CAD build for the part. Positions are in the model's coordinates, mm. Give positions to 0.01 mm unless a question says otherwise; leave off trailing zeros. Write each loop counter-clockwise with the first axis right and the second up, starting at its lowest first coordinate (ties: lowest second). Pieces come first, ordered by that corner, then holes. Notation, with made-up numbers: M 22,-28 L 80,-28 A18 ccw 80,-21 Z; hole C 7.5,69 d7. An arc over 180 degrees is marked long. One line per question, with ' | ' between items. Start each with the question number.
1. Flat gauge pin, fed straight in: pin 1 (3 mm diameter, centred on x = -38.1, z = 247.65, fed in from -Y). Where does the tip first touch, or does it go through?
2. Wall check: L1, parallel to Z at x = 25.5, y = 5; L2, parallel to Z at x = 12.7, y = 3.75; L3, parallel to Z at x = 8.5, y = 3. Give the ranges that are in metal, low to high.
3. Cut at A-A, the plane z = 107.95. Write the cut outline in (x, y), then the cut area to 3 significant figures.
4. Cut at B-B, the plane y = 3. Count the separate pieces of the cut face and the enclosed holes in it, then the cut area to 3 significant figures.
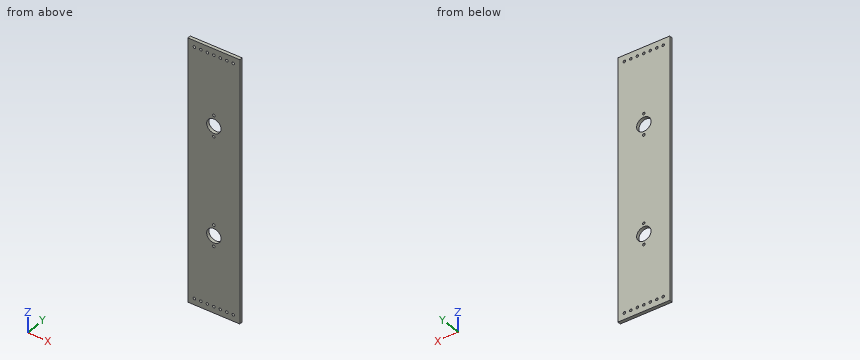
Autodesk Inventor part; units mm, degrees
ref_plane "YZ Plane" through (0, 0, 0) normal (1, 0, 0) x (0, 1, 0)
ref_plane "XZ Plane" through (0, 0, 0) normal (0, 1, 0) x (-1, 0, 0)
ref_plane "XY Plane" through (0, 0, 0) normal (0, 0, 1) x (1, 0, 0)
sketch "Sketch1" plane through (0, 0, 0) normal (0, 1, 0) x (-1, 0, 0)
  line L0 (-50.8, -260.35) -> (50.8, -260.35)
  line L1 (50.8, -260.35) -> (50.8, 260.35)
  line L2 (50.8, 260.35) -> (-50.8, 260.35)
  line L3 (-50.8, 260.35) -> (-50.8, -260.35)
  line L4 (-50.8, -260.35) -> (50.8, 260.35) construction
  line L5 (50.8, -260.35) -> (-50.8, 260.35) construction
  point P0 (0, 0)
  dimension "d0" = 101.6
  dimension "d1" = 520.7
extrude "Extrusion1" add sketch "Sketch1" along normal blind 6.35
sketch "Sketch2" plane through (0, 6.35, 0) normal (0, 1, 0) x (1, 0, 0)
  circle A0 centre (0, -107.95) radius 14.097
  circle A1 centre (0, 107.95) radius 14.097
  line L0 (0, -107.95) -> (0, 107.95) construction
  circle A2 centre (0, -107.95) radius 63.5 construction
  circle A3 centre (0, 107.95) radius 63.5 construction
  circle A4 centre (-107.4015, 0) radius 57.15 construction
  circle A5 centre (0, 44.5491) radius 14.097
  point P0 (0, 0)
  point P1 (0, 0)
  point P2 (0, -44.45)
  point P3 (0, 44.45)
  dimension "d7" = 127
  dimension "d8" = 127
  dimension "d5" = 28.194
  dimension "d9" = 88.9
  dimension "d10" = 114.3
  dimension "d12" = 152.4991
extrude "Extrusion2" cut sketch "Sketch2" against normal blind 6.35 contours A0 | A1
sketch "Sketch3" plane through (0, 6.35, 0) normal (0, 1, 0) x (1, 0, 0)
  line L0 (-50.8, -260.35) -> (50.8, -260.35)
  line L1 (-50.8, 260.35) -> (-50.8, -260.35)
  line L2 (-50.8, 260.35) -> (-50.8, -260.35) construction
  line L3 (-50.8, 0) -> (50.8, 0) construction
  line L4 (50.8, -260.35) -> (50.8, 260.35) construction
  point P0 (0, 0)
  point P1 (-38.1, -247.65)
  point P2 (-25.4, -247.65)
  point P3 (-12.7, -247.65)
  point P4 (0, -247.65)
  point P5 (12.7, -247.65)
  point P6 (25.4, -247.65)
  point P7 (38.1, -247.65)
  point P8 (-38.1, 247.65)
  point P9 (-25.4, 247.65)
  point P10 (-12.7, 247.65)
  point P11 (0, 247.65)
  point P12 (12.7, 247.65)
  point P13 (25.4, 247.65)
  point P14 (38.1, 247.65)
  dimension "d15" = 12.7
  dimension "d16" = 12.7
  dimension "d19" = 12.7
hole "Hole1" at (-38.1, 6.35, 247.65) at (-25.4, 6.35, 247.65) at (-12.7, 6.35, 247.65) at (0, 6.35, 247.65) at (12.7, 6.35, 247.65) at (25.4, 6.35, 247.65) at (38.1, 6.35, 247.65) at (38.1, 6.35, -247.65) at (25.4, 6.35, -247.65) at (12.7, 6.35, -247.65) at (0, 6.35, -247.65) at (-12.7, 6.35, -247.65) at (-25.4, 6.35, -247.65) at (-38.1, 6.35, -247.65) direction (0, -1, 0) diameter 5.1054 end through all
sketch "Sketch4" plane through (0, 6.35, 0) normal (0, 1, 0) x (1, 0, 0)
  line L0 (0, -86.9315) -> (0, -128.9685) construction
  line L1 (0, 128.9685) -> (0, 86.9315) construction
  circle A0 centre (-25.4, 247.65) radius 2.5527
  circle A1 centre (0, 247.65) radius 2.5527
  circle A2 centre (25.4, 247.65) radius 2.5527
  circle A3 centre (38.1, -247.65) radius 2.5527
  circle A4 centre (12.7, -247.65) radius 2.5527
  circle A5 centre (-12.7, -247.65) radius 2.5527
  circle A6 centre (-38.1, -247.65) radius 2.5527
  circle A7 centre (-25.4, -247.65) radius 2.5527
  circle A8 centre (0, -247.65) radius 2.5527
  circle A9 centre (25.4, -247.65) radius 2.5527
  circle A10 centre (38.1, 247.65) radius 2.5527
  circle A11 centre (12.7, 247.65) radius 2.5527
  circle A12 centre (-12.7, 247.65) radius 2.5527
  circle A13 centre (-38.1, 247.65) radius 2.5527
  circle A14 centre (0, 107.95) radius 14.097
  circle A15 centre (0, -107.95) radius 14.097
  line L2 (-50.8, 260.35) -> (50.8, 260.35)
  line L3 (50.8, 260.35) -> (50.8, -260.35)
  line L4 (50.8, -260.35) -> (-50.8, -260.35)
  line L5 (-50.8, -260.35) -> (-50.8, 260.35)
  point P0 (0, 0)
  dimension "d31" = 42.037
  dimension "d32" = 42.037
hole "Hole2" at (0, 6.35, -128.9685) at (0, 6.35, -86.9315) at (0, 6.35, 86.9315) at (0, 6.35, 128.9685) direction (0, -1, 0) diameter 5.1054 end through all
properties part number "GI - 007" material "Aluminum 6061"
Here are the results:
1) pin 1: through
2) L1: -260.35 to -250.2, -245.1 to 245.1, 250.2 to 260.35 | L2: -260.35 to -250.2, -245.1 to -114.07, -101.83 to 101.83, 114.07 to 245.1, 250.2 to 260.35 | L3: -260.35 to -119.2, -96.7 to 96.7, 119.2 to 260.35
3) outline: M -50.8,0 L -14.1,0 L -14.1,6.35 L -50.8,6.35 Z; M 14.1,0 L 50.8,0 L 50.8,6.35 L 14.1,6.35 Z | area: 466 mm^2
4) separate pieces: 1 | enclosed holes: 20 | area: 51,300 mm^2
